Build history of the part. All positions in model axes, mm. Face numbers are marked on the shaded views. A direction names the side the tool comes from. Round coordinates to 2 decimals unless told otherwise and drop trailing zeros. Write each loop counter-clockwise with the first axis right and the second up, starting at its lowest first coordinate (ties: lowest second). Pieces come first, ordered by that corner, then holes. Notation, with made-up numbers: M -4,4.25 L 4,4.25 A23 ccw 4,22.25 Z; hole C 53.5,75 d8. An arc over 180 degrees is marked long. Use a Markdown table: item, result.
from build123d import *

# Parameters (mm, degrees)
PAD_DEPTH           = 5
PAD_DEPTH_BACK      = 1
SKETCH001_W         = 14.05
SKETCH001_H         = 14.05
POCKET_DEPTH        = 1.001
POCKET_DEPTH_BACK   = 5.001
SKETCH004_W         = 4
SKETCH004_H         = 18
POCKET002_DEPTH     = 3.5
LINEARPATTERN_COUNT = 6
LINEARPATTERN_PITCH = 19.05
POCKET001_DEPTH     = 1.001
SKETCH005_R         = 1.35
PAD001_DEPTH        = 5
PAD001_DEPTH_BACK   = 1
CHAMFER_SIZE        = 1
SKETCH006_W         = 20.77
SKETCH006_H         = 18.64
POCKET003_DEPTH     = 4
SKETCH007_W         = 12
SKETCH007_H         = 1
SKETCH007_W_2       = 4
POCKET004_DEPTH     = 3
SKETCH008_W         = 27.2
SKETCH008_H         = 28
POCKET005_DEPTH     = 1.001


with BuildPart() as part:
    # Sketch → Pad (new body, two sides)
    with BuildSketch(Plane.XY) as pad_sk:
        with BuildLine():
            Line((-45.5, 11), (-45.5, -11))
            ThreePointArc((-45.5, -11), (-45.207107, -11.707107), (-44.5, -12))
            Line((-44.5, -12), (107, -12))
            ThreePointArc((107, -12), (107.707107, -11.707107), (108, -11))
            Line((108, 11), (108, -11))
            ThreePointArc((108, 11), (107.707107, 11.707107), (107, 12))
            Line((-44.5, 12), (107, 12))
            ThreePointArc((-44.5, 12), (-45.207107, 11.707107), (-45.5, 11))
        make_face()
    extrude(amount=PAD_DEPTH)
    extrude(pad_sk.sketch, amount=-PAD_DEPTH_BACK)

    # Sketch001 → Pocket (cut, two sides)
    with BuildSketch(Plane.XY) as pocket_sk:
        Rectangle(SKETCH001_W, SKETCH001_H)
    pocket = extrude(amount=-POCKET_DEPTH, mode=Mode.SUBTRACT) + extrude(pocket_sk.sketch, amount=POCKET_DEPTH_BACK, mode=Mode.SUBTRACT)

    # Sketch004 → Pocket002 (cut)
    with BuildSketch(Plane.XY):
        Rectangle(SKETCH004_W, SKETCH004_H)
    pocket002 = extrude(amount=POCKET002_DEPTH, mode=Mode.SUBTRACT)

    # LinearPattern: Pocket, Pocket002 ×6
    with Locations(*[(i * LINEARPATTERN_PITCH, 0, 0) for i in range(1, LINEARPATTERN_COUNT)]):
        add(pocket, mode=Mode.SUBTRACT)
        add(pocket002, mode=Mode.SUBTRACT)

    # Sketch002 → Pocket001 (cut, through all)
    with BuildSketch(Plane.XY):
        with BuildLine():
            Line((-43.6, 9.1), (-43.6, -9.1))
            ThreePointArc((-43.6, -9.1), (-43.307107, -9.807107), (-42.6, -10.1))
            Line((-42.6, -10.1), (104.1, -10.1))
            ThreePointArc((104.1, -10.1), (104.807107, -9.807107), (105.1, -9.1))
            Line((105.1, 9.1), (105.1, -9.1))
            ThreePointArc((105.1, 9.1), (104.807107, 9.807107), (104.1, 10.1))
            Line((-42.6, 10.1), (104.1, 10.1))
            ThreePointArc((-42.6, 10.1), (-43.307107, 9.807107), (-43.6, 9.1))
        make_face()
    extrude(amount=-POCKET001_DEPTH, mode=Mode.SUBTRACT)

    # Sketch005 → Pad001 (join, two sides)
    with BuildSketch(Plane.XY) as pad001_sk:
        with BuildLine():
            Line((65.473721, 12), (84.526279, 12))
            ThreePointArc((77.165064, 16.25), (80.276279, 13.138784), (84.526279, 12))
            ThreePointArc((77.165064, 16.25), (75, 17.5), (72.834936, 16.25))
            ThreePointArc((65.473721, 12), (69.723721, 13.138784), (72.834936, 16.25))
        make_face()
        with Locations((75, 15)):
            Circle(SKETCH005_R, mode=Mode.SUBTRACT)
        with BuildLine():
            Line((-14.526279, 12), (4.526279, 12))
            ThreePointArc((-2.834936, 16.25), (0.276279, 13.138784), (4.526279, 12))
            ThreePointArc((-2.834936, 16.25), (-5, 17.5), (-7.165064, 16.25))
            ThreePointArc((-14.526279, 12), (-10.276279, 13.138784), (-7.165064, 16.25))
        make_face()
        with Locations((-5, 15)):
            Circle(SKETCH005_R, mode=Mode.SUBTRACT)
    pad001 = extrude(amount=PAD001_DEPTH) + extrude(pad001_sk.sketch, amount=-PAD001_DEPTH_BACK)

    # Mirrored: Pad001 across XZ
    add(pad001.mirror(Plane.XZ))

    # Chamfer
    chamfer_edges = [part.edges().sort_by_distance(p)[0] for p in [
        (73.65, 15, 5),
        (-6.35, 15, 5),
        (-6.35, -15, 5),
        (73.65, -15, 5),
    ]]
    chamfer(chamfer_edges, length=CHAMFER_SIZE)

    # Sketch006 → Pocket003 (cut)
    with BuildSketch(Plane.XY):
        with Locations((-33.035, 0)):
            Rectangle(SKETCH006_W, SKETCH006_H)
    extrude(amount=POCKET003_DEPTH, mode=Mode.SUBTRACT)

    # Sketch007 → Pocket004 (cut)
    with BuildSketch(Plane.XY):
        with Locations((-17, -8)):
            Rectangle(SKETCH007_W, SKETCH007_H)
        with Locations((85.5, -8)):
            Rectangle(SKETCH007_W_2, SKETCH007_H)
    extrude(amount=POCKET004_DEPTH, mode=Mode.SUBTRACT)

    # Sketch008 → Pocket005 (cut, through all)
    with BuildSketch(Plane.XY.offset(4)):
        with Locations((-22.5, 6)):
            Rectangle(SKETCH008_W, SKETCH008_H)
    extrude(amount=POCKET005_DEPTH, mode=Mode.SUBTRACT)


solid = part.part
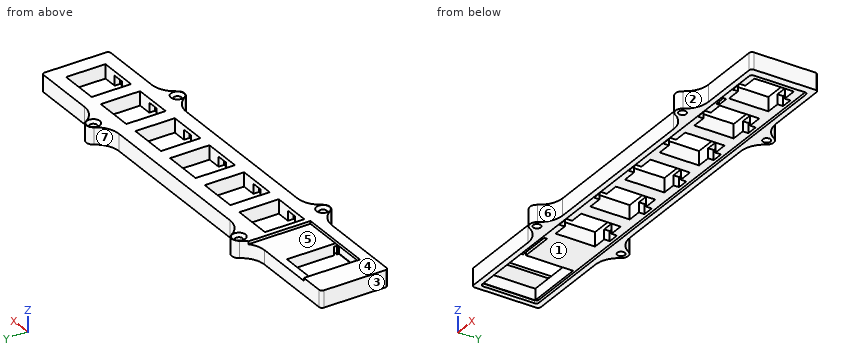
Q1. Which spindle directions (+Z, -Z, +X, -X, +Y, -Y) get a long thin tool onto all of the face, cutting with end or side? Do the marked faces 4, 5, 6 and 7. Say none if no direction does.
Response values:
| item | result |
|---|---|
| face 4 | +Z, +X, -X, +Y, -Y |
| face 5 | +Z, +Y |
| face 6 | +Z, -Z, -Y |
| face 7 | +Z, -Z, +Y |
Q2. Cut at A-A on x = -5. Give the cut face in (y, z) (3 decimals).
Response values:
| item | result |
|---|---|
| outline | M -17.5,-1 L -16.35,-1 L -16.35,4 L -17.35,5 L -17.5,5 Z; M -13.65,-1 L -10.1,-1 L -10.1,0 L -7.025,0 L -7.025,5 L -12.65,5 L -13.65,4 Z; M 7.025,0 L 10.1,0 L 10.1,-1 L 13.65,-1 L 13.65,4 L 12.65,5 L 7.025,5 Z; M 16.35,-1 L 17.5,-1 L 17.5,5 L 17.35,5 L 16.35,4 Z |
Q3. Two-plate mould, pull along Y, no slides. Class the marked faces 1, 2 and 3: +Y half, -Y half, draft (parallel to the pull), parting line (faces both ways), or undercut.
Response values:
| item | result |
|---|---|
| face 1 | undercut |
| face 2 | -Y half |
| face 3 | draft |
Q4. Drill centre lines: L1, parallel to Y at x = -5, z = 1.75 (3 decimals); L2, parallel to Y at x = 25, z = 3.55 (3 decimals); L3, parallel to Y at x = 75, z = 0.15. Where is each one in solid material? Low to high.
Response values:
| item | result |
|---|---|
| L1 | y = -17.5 to -16.35, -13.65 to -7.025, 7.025 to 13.65, 16.35 to 17.5 |
| L2 | y = -12 to -7.025, 7.025 to 12 |
| L3 | y = -17.5 to -16.35, -13.65 to -9, 9 to 13.65, 16.35 to 17.5 |
Q5. Cut at C-C on y = 1.5. Count the separate pieces of the cut face and the enclosed holes in it, and give its area (3 significant figures).
Response values:
| item | result |
|---|---|
| separate pieces | 8 |
| enclosed holes | 0 |
| area | 241 mm2 |
Q6. Drop flat-ended pins along their axis: P1, Ø2.5, axis at x = 39.5, z = 2.5, coming from the -Y side; P2, Ø2, axis at x = 95, y = -8.5, coming from the -Z side; P3, Ø2.5, axis at x = 55.5, z = 3, coming from the +Y side. Give the stop position or say it passes through.
Response values:
| item | result |
|---|---|
| P1 | stops at y = -12 |
| P2 | stops at z = 0 |
| P3 | stops at y = 12 |
Q7. Cut at B-B on x = 62. Give the cut face in (y, z) (3 decimals), and give its area (4 significant figures).
Response values:
| item | result |
|---|---|
| outline | M -12,-1 L -10.1,-1 L -10.1,0 L -7.025,0 L -7.025,5 L -12,5 Z; M 7.025,0 L 10.1,0 L 10.1,-1 L 12,-1 L 12,5 L 7.025,5 Z |
| area | 53.55 mm2 |
